```python
from build123d import *

# Parameters (mm, degrees)
SKETCH1_R           = 45
SKETCH1_R_2         = 20
BOSS_EXTRUDE1_DEPTH = 30
CUT_EXTRUDE1_DEPTH  = 30


with BuildPart() as part:
    # Sketch1 → Boss-Extrude1 (new body)
    with BuildSketch(Plane.XY):
        Circle(SKETCH1_R)
        Circle(SKETCH1_R_2, mode=Mode.SUBTRACT)
    extrude(amount=BOSS_EXTRUDE1_DEPTH)

    # Sketch2 → Cut-Extrude1 (cut)
    with BuildSketch(Plane.XY.offset(30)):
        with BuildLine():
            Line((-24.907553239, 26.610521963), (-18.211403795, 23.452988079))
            ThreePointArc((-18.211403795, 23.452988079), (-14.122579745, 22.499392212), (-10.002690574, 23.308305316))
            ThreePointArc((-10.002690574, 23.308305316), (-4.902050675, 24.885755255), (0.415790578, 25.360560594))
            ThreePointArc((0.415790578, 25.360560594), (4.483384622, 26.152621175), (7.880614817, 28.525701089))
            Line((7.880614817, 28.525701089), (13.020947118, 34.017606823))
            ThreePointArc((13.020947118, 34.017606823), (13.72723623, 36.848657497), (11.693481002, 38.940912716))
            ThreePointArc((11.693481002, 38.940912716), (-7.808912198, 39.901792835), (-25.510313511, 31.660007671))
            ThreePointArc((-25.510313511, 31.660007671), (-26.606889428, 28.968389927), (-24.907553239, 26.610521963))
        make_face()
        with BuildLine():
            Line((28.525701089, -7.880614817), (34.017606823, -13.020947118))
            ThreePointArc((34.017606823, -13.020947118), (36.848657497, -13.72723623), (38.940912716, -11.693481002))
            ThreePointArc((38.940912716, -11.693481002), (39.901792835, 7.808912198), (31.660007671, 25.510313511))
            ThreePointArc((31.660007671, 25.510313511), (28.968389927, 26.606889428), (26.610521963, 24.907553239))
            Line((26.610521963, 24.907553239), (23.452988079, 18.211403795))
            ThreePointArc((23.452988079, 18.211403795), (22.499392212, 14.122579745), (23.308305316, 10.002690574))
            ThreePointArc((23.308305316, 10.002690574), (24.885755255, 4.902050675), (25.360560594, -0.415790578))
            ThreePointArc((25.360560594, -0.415790578), (26.152621175, -4.483384622), (28.525701089, -7.880614817))
        make_face()
        with BuildLine():
            Line((-7.880614817, -28.525701089), (-13.020947118, -34.017606823))
            ThreePointArc((-13.020947118, -34.017606823), (-13.72723623, -36.848657497), (-11.693481002, -38.940912716))
            ThreePointArc((-11.693481002, -38.940912716), (7.808912198, -39.901792835), (25.510313511, -31.660007671))
            ThreePointArc((25.510313511, -31.660007671), (26.606889428, -28.968389927), (24.907553239, -26.610521963))
            Line((24.907553239, -26.610521963), (18.211403795, -23.452988079))
            ThreePointArc((18.211403795, -23.452988079), (14.122579745, -22.499392212), (10.002690574, -23.308305316))
            ThreePointArc((10.002690574, -23.308305316), (4.902050675, -24.885755255), (-0.415790578, -25.360560594))
            ThreePointArc((-0.415790578, -25.360560594), (-4.483384622, -26.152621175), (-7.880614817, -28.525701089))
        make_face()
        with BuildLine():
            Line((-28.525701089, 7.880614817), (-34.017606823, 13.020947118))
            ThreePointArc((-34.017606823, 13.020947118), (-36.848657497, 13.72723623), (-38.940912716, 11.693481002))
            ThreePointArc((-38.940912716, 11.693481002), (-39.901792835, -7.808912198), (-31.660007671, -25.510313511))
            ThreePointArc((-31.660007671, -25.510313511), (-28.968389927, -26.606889428), (-26.610521963, -24.907553239))
            Line((-26.610521963, -24.907553239), (-23.452988079, -18.211403795))
            ThreePointArc((-23.452988079, -18.211403795), (-22.499392212, -14.122579745), (-23.308305316, -10.002690574))
            ThreePointArc((-23.308305316, -10.002690574), (-24.885755255, -4.902050675), (-25.360560594, 0.415790578))
            ThreePointArc((-25.360560594, 0.415790578), (-26.152621175, 4.483384622), (-28.525701089, 7.880614817))
        make_face()
    extrude(amount=-CUT_EXTRUDE1_DEPTH, mode=Mode.SUBTRACT)


solid = part.part
```
Here's how the part is built. I have some questions about the finished solid (model axes, mm). Round coordinates to 2 decimals unless told otherwise and drop trailing zeros. Write each loop counter-clockwise with the first axis right and the second up, starting at its lowest first coordinate (ties: lowest second). Pieces come first, ordered by that corner, then holes.
Q1. Please list where these lines run through material, in increasing order: probe 1 along Y at (x, z) = (0, 15); probe 2 along X at (y, z) = (12, 18.75); probe 3 along X at (y, z) = (-6.5, 6.25).
Q2. Will these pins go through, and if not, where does the flat tip stop? P1, Ø2, axis at x = 33.5, z = 24, coming from the -Y side; P2, Ø2, axis at y = 13.5, z = 10, coming from the +X side; P3, Ø8, axis at y = -26, z = 16, coming from the +X side.
Q3. If we section it at B-B on z = 9.5: Give the number of separate pieces and of enclosed holes in the cut face, plus the area to 3 significant figures.
Q4. If we section it at A-A on y = -16: Write out the boundary of the cut face in (x, z), plus the area to 3 significant figures.
Q5. If we mould it in two halves opening along X, with no side actions, what happens to faces 1 (the cylindrical face through (36.807, -13.738, 15.21)), 2 (the cylindrical face through (4.98, -24.87, 15.21))? For each: +X half, -X half, draft (parallel to the pull), parting line (faces both ways), or undercut.
Answer below:
1. probe 1: y = -45 to -40.66, -25.36 to -20, 20 to 25.36, 40.66 to 45
1. probe 2: x = -43.37 to -38.83, -32.93 to -16, 16 to 22.69, 38.85 to 43.37
1. probe 3: x = -44.53 to -40.14, -24.52 to -18.91, 18.91 to 27.3, 40.14 to 44.53
2. P1: stops at y = -31.12
2. P2: stops at x = 43.23
2. P3: stops at x = 39.26
3. separate pieces: 1
3. enclosed holes: 5
3. area: 3,090 mm2
4. outline: (-42.06, 0) - (-37.38, 0) - (-37.38, 30) - (-42.06, 30) - close; (-22.71, 0) - (-12, 0) - (-12, 30) - (-22.71, 30) - close; (12, 0) - (42.06, 0) - (42.06, 30) - (12, 30) - close
4. area: 1,360 mm2
5. face 1: undercut
5. face 2: undercut
